Autodesk Fusion 360 part; units mm, degrees
sketch "Sketch1" plane through (0, 0, 0) normal (0, 1, 0) x (1, 0, 0)
  line L0 (-190, 118.3432) -> (-10, 118.3432)
  line L1 (0, 108.3432) -> (0, 10)
  line L2 (-10, 0) -> (-190, 0)
  line L3 (-200, 10) -> (-200, 108.3432)
  arc A0 (-190, 118.3432) -> (-200, 108.3432) centre (-190, 108.3432) ccw
  arc A1 (-200, 10) -> (-190, 0) centre (-190, 10) ccw
  arc A2 (-10, 0) -> (0, 10) centre (-10, 10) ccw
  arc A3 (0, 108.3432) -> (-10, 118.3432) centre (-10, 108.3432) ccw
  arc A4 (-3, 108.3432) -> (-10, 115.3432) centre (-10, 108.3432) ccw
  line L4 (-190, 115.3432) -> (-10, 115.3432)
  arc A5 (-190, 115.3432) -> (-197, 108.3432) centre (-190, 108.3432) ccw
  line L5 (-197, 10) -> (-197, 108.3432)
  arc A6 (-197, 10) -> (-190, 3) centre (-190, 10) ccw
  line L6 (-10, 3) -> (-190, 3)
  arc A7 (-10, 3) -> (-3, 10) centre (-10, 10) ccw
  line L7 (-3, 108.3432) -> (-3, 10)
  dimension "d3" = 200
  dimension "d4" = 118.3432
  dimension "d6" = 10
  dimension "d7" = 10
  dimension "d8" = 10
  dimension "d9" = 10
  dimension "d15" = 3
extrude "Extrude2" add sketch "Sketch1" along normal blind 3 contours L0 L1 L2 L3 A0 A1 A2 A3 | A4 L4 A5 L5 A6 L6 A7 L7 makes body 1
extrude "Extrude3" add sketch "Sketch1" along normal blind 30 separate body makes body 2
combine "Combine1" operation add target body 2 tool bodies 1
sketch "Sketch2" plane through (0, 0, 0) normal (0, 0, 1) x (1, 0, 0)
  line L0 (-10, 0) -> (-10, 30)
  line L1 (-10, 30) -> (-190, 30)
  line L2 (-190, 30) -> (-190, 0)
  line L3 (-190, 0) -> (-10, 0)
  line L4 (-100, 30) -> (-100, 0)
  line L5 (-10, 30) -> (-10, 50)
  line L6 (-30, 50) -> (-30, 43)
  line L7 (-30, 43) -> (-65.7143, 30)
  line L8 (-10, 30) -> (-65.7143, 30)
  line L9 (-30, 50) -> (-30, 51)
  arc A0 (-10, 50) -> (-30, 51) centre (-19.975, 51) ccw
  circle A1 centre (-19.975, 51) radius 1.975
  line L10 (-170, 43) -> (-134.2857, 30)
  line L11 (-190, 30) -> (-134.2857, 30)
  line L12 (-190, 30) -> (-190, 50)
  arc A2 (-170, 51) -> (-190, 50) centre (-180.025, 51) ccw
  line L13 (-170, 50) -> (-170, 43)
  line L14 (-170, 50) -> (-170, 51)
  circle A3 centre (-180.025, 51) radius 1.975
extrude "Extrude4" add sketch "Sketch2" against normal blind 3 contours L1 L5 L6 L7 L8 L9 A0 | L1 L10 L11 L12 A2 L13 L14 bodies 2
equation "leveys = 200 mm"
equation "d3 = leveys"
equation "d4 = leveys / 1.69"
equation "fillet = 10 mm"
equation "d6 = fillet"
equation "d7 = fillet"
equation "d8 = fillet"
equation "d9 = fillet"
equation "paksuus = 30 mm"
equation "pohjanpaksuus = 3 mm"
equation "reuna = 3 mm"
equation "d15 = reuna"
equation "d16 = pohjanpaksuus"
equation "d18 = paksuus"
Here's how the part is built. I have some questions about the finished solid (model axes, mm). A direction names the side the tool comes from. Round coordinates to 2 decimals unless told otherwise and drop trailing zeros. Loops run counter-clockwise (first coordinate to the right, second up) from the corner with the lowest first, then second, coordinate; pieces in that order, holes last.
1. Thinking about a two-plate mould opening in X: for faces 4 (the face through (-196.99, 14.79, -2.85)), 5 (the face through (-2.85, 14.79, -3.01)), 6 (the face through (-3, 16, -60)), which applies, released by +X, released by -X, zero draft, split by the parting line, or undercut?
Answers:
face 4: released by -X
face 5: released by +X
face 6: undercut
2. Suppose I cut it at B-B, the plane z = -21. Please give me the cut outline in (x, y), and give its area (3 significant figures).
Answers:
outline: (-200, 0) - (0, 0) - (0, 30) - (-3, 30) - (-3, 3) - (-197, 3) - (-197, 30) - (-200, 30) - close
area: 762 mm2
3. Will these pins go through, and if not, where does the flat tip stop? pin 1 (1.5 mm diameter, centred on y = 35.5, z = -1, fed in from -X); pin 2 (6 mm diameter, centred on x = -135.5, z = -96.5, fed in from -Y); pin 3 (3.5 mm diameter, centred on x = -19.975, y = 51, fed in from +Z); pin 4 (2.5 mm diameter, centred on y = 47.5, z = -2, fed in from +X).
Answers:
pin 1: stops at x = -190
pin 2: stops at y = 0
pin 3: passes through
pin 4: stops at x = -10
4. If I drill on probe 1 along Z at (x, y) = (-86, 29); probe 2 along X at (y, z) = (27.5, -25.5); probe 3 along Z at (x, y) = (-187, 57), over which ranges is the centre line in solid material (lowest first)?
Answers:
probe 1: z = -118.34 to -115.34, -3 to 0
probe 2: x = -200 to -197, -3 to 0
probe 3: z = -3 to 0
5. For faces 1 (the face through (-5.105, 16.311, -113.347)), 2 (the face through (-101, 15, -118.343)), 3 (the face through (-47.61, 36.59, -1.48)), which set-ups out of +Z, -Z, +X, -X, +Y, -Y let a thin tool reach every point of the face, with its end or its side?
Answers:
face 1: +Y
face 2: -Z, +X, -X, +Y, -Y
face 3: +Z, -Z, +Y
6. Suppose I cut it at D-D, the plane x = -131.5. Please give me the cut outline in (y, z), and give its area (3 significant figures).
Answers:
outline: (0, -118.34) - (30, -118.34) - (30, -115.34) - (3, -115.34) - (3, -3) - (30, -3) - (30, 0) - (0, 0) - close
area: 517 mm2
7. Suppose I cut it at C-C, the plane y = 41. Please give me the cut outline in (x, z).
Answers:
outline: (-190, -3) - (-164.51, -3) - (-164.51, 0) - (-190, 0) - close; (-35.49, -3) - (-10, -3) - (-10, 0) - (-35.49, 0) - close
8. Suppose I cut it at A-A, the plane y = 12.5. Please give me the cut outline in (x, z).
Answers:
outline: (-200, -108.34) arc R10 ccw to (-190, -118.34) - (-10, -118.34) arc R10 ccw to (0, -108.34) - (0, -10) arc R10 ccw to (-10, 0) - (-190, 0) arc R10 ccw to (-200, -10) - close; hole (-197, -108.34) arc R7 ccw to (-190, -115.34) - (-10, -115.34) arc R7 ccw to (-3, -108.34) - (-3, -10) arc R7 ccw to (-10, -3) - (-190, -3) arc R7 ccw to (-197, -10) - close
